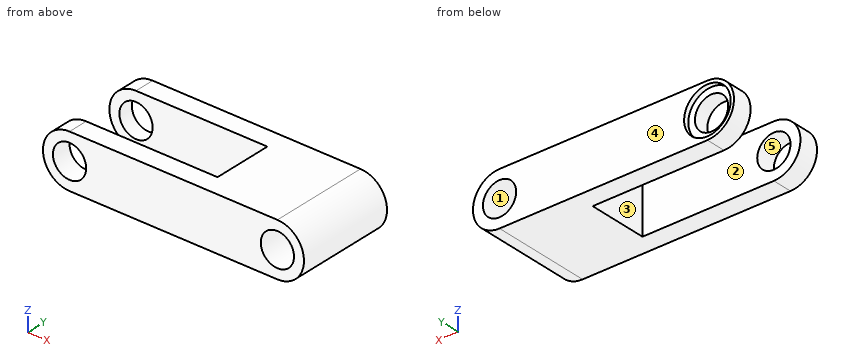
```python
from build123d import *

# Parameters (mm, degrees)
EXTRUDE_1_DEPTH     = 60
CUT_EXTRUDE_1_REACH = 102.091
SKETCH_2_R          = 10
CUT_EXTRUDE_2_REACH = 102.091
SKETCH_3_R          = 10
SKETCH_4_R          = 14
CUT_EXTRUDE_3_DEPTH = 3
CUT_EXTRUDE_4_REACH = 105.857
SKETCH_6_W          = 115
SKETCH_6_H          = 36


with BuildPart() as part:
    # Sketch 1 → Extrude 1 (new body)
    with BuildSketch(Plane(origin=(0, 0, 0), x_dir=(1, 0, 0), z_dir=(0, 1, 0))):
        with BuildLine():
            Line((-62.5, 16), (62.5, 16))
            ThreePointArc((62.5, 16), (78.5, 0), (62.5, -16))
            Line((62.5, -16), (-62.5, -16))
            ThreePointArc((-62.5, -16), (-78.5, 0), (-62.5, 16))
        make_face()
    extrude(amount=EXTRUDE_1_DEPTH)

    # Sketch 2 → Cut-Extrude 1 (cut, up to next)
    with BuildSketch(Plane(origin=(0, 60, 0), x_dir=(1, 0, 0), z_dir=(0, 1, 0)), mode=Mode.PRIVATE) as cut_extrude_1_sk1:
        with Locations(Location((62.5, 0, 0), (0, 0, 270))):
            Circle(SKETCH_2_R)
    cut_extrude_1_tool1 = extrude(cut_extrude_1_sk1.sketch, amount=-CUT_EXTRUDE_1_REACH, mode=Mode.PRIVATE) & part.part
    add(cut_extrude_1_tool1.solids().sort_by_distance((62.5, 60, 0))[0], mode=Mode.SUBTRACT)

    # Sketch 3 → Cut-Extrude 2 (cut, up to next)
    with BuildSketch(Plane(origin=(0, 60, 0), x_dir=(1, 0, 0), z_dir=(0, 1, 0)), mode=Mode.PRIVATE) as cut_extrude_2_sk1:
        with Locations(Location((-62.5, 0, 0), (0, 0, 270))):
            Circle(SKETCH_3_R)
    cut_extrude_2_tool1 = extrude(cut_extrude_2_sk1.sketch, amount=-CUT_EXTRUDE_2_REACH, mode=Mode.PRIVATE) & part.part
    add(cut_extrude_2_tool1.solids().sort_by_distance((-62.5, 60, 0))[0], mode=Mode.SUBTRACT)

    # Sketch 4 → Cut-Extrude 3 (cut)
    with BuildSketch(Plane(origin=(0, 60, 0), x_dir=(1, 0, 0), z_dir=(0, 1, 0))):
        with Locations(Location((-62.5, 0, 0), (0, 0, 270))):
            Circle(SKETCH_4_R)
    extrude(amount=-CUT_EXTRUDE_3_DEPTH, mode=Mode.SUBTRACT)

    # Sketch 6 → Cut-Extrude 4 (cut, up to next)
    with BuildSketch(Plane.XY.offset(16), mode=Mode.PRIVATE) as cut_extrude_4_sk1:
        with Locations((-41, 30)):
            Rectangle(SKETCH_6_W, SKETCH_6_H)
    cut_extrude_4_tool1 = extrude(cut_extrude_4_sk1.sketch, amount=-CUT_EXTRUDE_4_REACH, mode=Mode.PRIVATE) & part.part
    add(cut_extrude_4_tool1.solids().sort_by_distance((-41, 30, 16))[0], mode=Mode.SUBTRACT)


solid = part.part
```
The model under review builds one solid part; all positions refer to its coordinate system, in mm. Face numbers are marked on the shaded views. A direction names the side the tool comes from. Coordinates: 2 decimals unless noted, no trailing zeros. Order: outer loops, then holes, each group sorted by start corner. A loop starts at its lowest first (then second) coordinate and runs counter-clockwise, first axis right, second up. Notation, with made-up numbers: (25.25, 2) -> (53.25, 2) arc R15 ccw to (53.25, 20) -> close; hole circle Ø3 at (28, -15). An arc over 180 degrees is marked (long way). Answer in a Markdown table with one row per item. Add a question column.
Item 1: Machinability: for the marked faces 1 and 2, which of the approach directions +Z, -Z, +X, -X, +Y, -Y give a long, thin tool a straight path to every point of the face, cutting with its end or side? Answer none if there is none.
Item 2: We need section A-A on z = 0. Write out the cut boundary in (x, y), plus the area to 3 significant figures.
Item 3: To check wall thickness, follow probe 1 along X at (y, z) = (59.15, 0); probe 2 along Z at (x, y) = (-62, 58); probe 3 along Y at (x, z) = (-4, -5). State the ranges of each line that lie inside material, in increasing order.
Item 4: Clearance check with flat-ended pins moving along their axes: pin 1 (8 mm diameter, centred on y = 49, z = -6.5, fed in from +X); pin 2 (2 mm diameter, centred on y = 24.5, z = 5.5, fed in from +X); pin 3 (10 mm diameter, centred on x = -54.5, z = -1, fed in from +Y). State where each tip first meets the part, or that it passes through.
Item 5: We need section D-D on z = -8. Write out the cut boundary in (x, y), plus the area to 3 significant figures.
Item 6: Mouldability with a two-part tool opening along X and no side actions: class the marked faces 3, 4 and 5 as +X half, -X half, draft (parallel to the pull), parting line (faces both ways), or undercut.
Item 7: We need section B-B on x = -47. Write out the cut boundary in (y, z).
Item 8: We need section C-C on y = 42.5. Write out the cut boundary in (x, z).
Final values:
| question | item | result |
|---|---|---|
| 1 | face 1 | +Y, -Y |
| 1 | face 2 | +Z, -Z, -X |
| 2 | outline | (-78.5, 0) -> (-72.5, 0) -> (-72.5, 12) -> (-78.5, 12) -> close; (-78.5, 48) -> (-72.5, 48) -> (-72.5, 57) -> (-76.5, 57) -> (-76.5, 60) -> (-78.5, 60) -> close; (-52.5, 0) -> (52.5, 0) -> (52.5, 60) -> (-48.5, 60) -> (-48.5, 57) -> (-52.5, 57) -> (-52.5, 48) -> (16.5, 48) -> (16.5, 12) -> (-52.5, 12) -> close; (72.5, 0) -> (78.5, 0) -> (78.5, 60) -> (72.5, 60) -> close |
| 2 | area | 4,300 mm2 |
| 3 | probe 1 | x = -78.5 to -76.5, -48.5 to 52.5, 72.5 to 78.5 |
| 3 | probe 2 | z = -16 to -13.99, 13.99 to 16 |
| 3 | probe 3 | y = 0 to 12, 48 to 60 |
| 4 | pin 1 | stops at x = 78.3 |
| 4 | pin 2 | stops at x = 77.85 |
| 4 | pin 3 | stops at y = 57 |
| 5 | outline | (-76.36, 0) -> (-68.5, 0) -> (-68.5, 12) -> (-76.36, 12) -> close; (-76.36, 48) -> (-68.5, 48) -> (-68.5, 57) -> (-73.99, 57) -> (-73.99, 60) -> (-76.36, 60) -> close; (-56.5, 0) -> (56.5, 0) -> (56.5, 60) -> (-51.01, 60) -> (-51.01, 57) -> (-56.5, 57) -> (-56.5, 48) -> (16.5, 48) -> (16.5, 12) -> (-56.5, 12) -> close; (68.5, 0) -> (76.36, 0) -> (76.36, 60) -> (68.5, 60) -> close |
| 5 | area | 4,780 mm2 |
| 6 | face 3 | -X half |
| 6 | face 4 | draft |
| 6 | face 5 | undercut |
| 7 | outline | (0, -16) -> (12, -16) -> (12, 16) -> (0, 16) -> close; (48, -16) -> (60, -16) -> (60, 16) -> (48, 16) -> close |
| 8 | outline | (16.5, -16) -> (62.5, -16) arc R16 ccw to (62.5, 16) -> (16.5, 16) -> close; hole circle Ø20 at (62.5, 0) |
